```python
from build123d import *

# Parameters (mm, degrees)
SKETCH1_W                = 33.02
SKETCH1_H                = 10.16
SKETCH1_R                = 3
SKETCH1_R_2              = 1.7
BOSS_EXTRUDE1_DEPTH      = 1
SKETCH2_W                = 6
SKETCH2_H                = 1
SKETCH2_W_2              = 1
SKETCH2_H_2              = 6
BOSS_EXTRUDE2_DEPTH      = 6
SKETCH3_R                = 1
CUT_EXTRUDE1_DEPTH       = 21.610815122
FILLET1_R                = 1
BOSS_EXTRUDE3_DEPTH      = 1
BOSS_EXTRUDE3_DEPTH_BACK = 1


with BuildPart() as part:
    # Sketch1 → Boss-Extrude1 (new body)
    with BuildSketch(Plane(origin=(0, 0, 0), x_dir=(1, 0, 0), z_dir=(0, 1, 0))):
        Rectangle(SKETCH1_W, SKETCH1_H)
        with Locations(Location((0, 0, 0), (0, 0, 270))):
            Circle(SKETCH1_R, mode=Mode.SUBTRACT)
        with Locations(Location((-12.7, 0, 0), (0, 0, 270))):
            Circle(SKETCH1_R_2, mode=Mode.SUBTRACT)
    extrude(amount=BOSS_EXTRUDE1_DEPTH)

    # Sketch2 → Boss-Extrude2 (add)
    with BuildSketch(Plane(origin=(0, 1, 0), x_dir=(1, 0, 0), z_dir=(0, 1, 0))):
        with Locations((-12.7, 4.58)):
            Rectangle(SKETCH2_W, SKETCH2_H)
        with Locations((-12.7, -4.58)):
            Rectangle(SKETCH2_W, SKETCH2_H)
        with Locations((16.01, 0)):
            Rectangle(SKETCH2_W_2, SKETCH2_H_2)
    extrude(amount=BOSS_EXTRUDE2_DEPTH)

    # Sketch3 → Cut-Extrude1 (cut, through all)
    with BuildSketch(Plane.XY.offset(5.08)):
        with Locations((-12.7, 5)):
            Circle(SKETCH3_R)
    extrude(amount=-CUT_EXTRUDE1_DEPTH, mode=Mode.SUBTRACT)

    # Fillet1
    # the kernel refuses this fillet: 1 mm, written as the material it adds along each edge
    with BuildSketch(Plane(origin=(-15.7, 1, -4.08), x_dir=(-1, 0, 0), z_dir=(0, 0, -1))) as fillet1_piece_1:
        with BuildLine():
            CenterArc((1, 0.98178409), FILLET1_R, 180, 79.047215801)
            Line((0, 0.98178409), (0, 0))
            Line((0, 0), (0.81, 0))
        make_face()
    extrude(amount=1)
    with BuildSketch(Plane(origin=(-9.7, 1, -4.08), x_dir=(0, 0, 1), z_dir=(-1, 0, 0))) as fillet1_piece_2:
        with BuildLine():
            CenterArc((FILLET1_R, FILLET1_R), FILLET1_R, 180, 90)
            Line((0, FILLET1_R), (0, 0))
            Line((0, 0), (FILLET1_R, 0))
        make_face()
    extrude(amount=6)
    with BuildSketch(Plane(origin=(-9.7, 1, -5.08), x_dir=(1, 0, 0), z_dir=(0, 0, 1))) as fillet1_piece_3:
        with BuildLine():
            CenterArc((FILLET1_R, FILLET1_R), FILLET1_R, 180, 90)
            Line((0, FILLET1_R), (0, 0))
            Line((0, 0), (FILLET1_R, 0))
        make_face()
    extrude(amount=1)
    with BuildSketch(Plane(origin=(16.51, 1, -3), x_dir=(0, 0, -1), z_dir=(-1, 0, 0)), Plane(origin=(15.51, 1, 3), x_dir=(0, 0, 1), z_dir=(1, 0, 0)), Plane(origin=(-9.7, 1, 5.08), x_dir=(1, 0, 0), z_dir=(0, 0, -1))) as fillet1_piece_4:
        with BuildLine():
            CenterArc((FILLET1_R, -FILLET1_R), FILLET1_R, 90, 90)
            Line((0, -FILLET1_R), (0, 0))
            Line((0, 0), (FILLET1_R, 0))
        make_face()
    extrude(amount=1)
    with BuildSketch(Plane(origin=(-15.7, 1, 4.08), x_dir=(-1, 0, 0), z_dir=(0, 0, 1))) as fillet1_piece_5:
        with BuildLine():
            CenterArc((1, -0.98178409), FILLET1_R, 100.952784199, 79.047215801)
            Line((0, -0.98178409), (0, 0))
            Line((0, 0), (0.81, 0))
        make_face()
    extrude(amount=1)
    with BuildSketch(Plane(origin=(-9.7, 1, 4.08), x_dir=(0, 0, -1), z_dir=(-1, 0, 0))) as fillet1_piece_6:
        with BuildLine():
            CenterArc((FILLET1_R, -FILLET1_R), FILLET1_R, 90, 90)
            Line((0, -FILLET1_R), (0, 0))
            Line((0, 0), (FILLET1_R, 0))
        make_face()
    extrude(amount=6)
    with BuildSketch(Plane(origin=(-15.7, 1, -1.625539774), x_dir=(-1, 0, 0), z_dir=(0, 0, -1))) as fillet1_piece_7a_section:
        with BuildLine():
            CenterArc((1, 0.98178409), FILLET1_R, 180, 79.047215801)
            Line((0, 0.98178409), (0, 0))
            Line((0, 0), (0.81, 0))
        make_face()
    fillet1_piece_7a = extrude(amount=3.454460226, mode=Mode.PRIVATE)
    fillet1_piece_7a = split(fillet1_piece_7a, bisect_by=Plane(origin=(-15.7, 1, -4.08), z_dir=(0, 0, 1)), keep=Keep.TOP, mode=Mode.PRIVATE)
    with BuildSketch(Plane(origin=(-9.7, 1, -4.08), x_dir=(0, 0, 1), z_dir=(-1, 0, 0))) as fillet1_piece_7b_section:
        with BuildLine():
            CenterArc((FILLET1_R, FILLET1_R), FILLET1_R, 180, 90)
            Line((0, FILLET1_R), (0, 0))
            Line((0, 0), (FILLET1_R, 0))
        make_face()
    fillet1_piece_7b = extrude(amount=8.5, mode=Mode.PRIVATE)
    fillet1_piece_7b = split(fillet1_piece_7b, bisect_by=Plane(origin=(-16.51, 1, -4.08), z_dir=(1, 0, 0)), keep=Keep.TOP, mode=Mode.PRIVATE)
    fillet1_piece_7b = split(fillet1_piece_7b, bisect_by=Plane(origin=(-15.7, 1, -4.08), z_dir=(-1, 0, 0)), keep=Keep.TOP, mode=Mode.PRIVATE)
    fillet1_piece_7 = fillet1_piece_7a & fillet1_piece_7b
    add(fillet1_piece_7)
    with BuildSketch(Plane(origin=(-7.2, 1, -4.08), x_dir=(0, 0, 1), z_dir=(-1, 0, 0))) as fillet1_piece_8a_section:
        with BuildLine():
            CenterArc((FILLET1_R, FILLET1_R), FILLET1_R, 180, 90)
            Line((0, FILLET1_R), (0, 0))
            Line((0, 0), (FILLET1_R, 0))
        make_face()
    fillet1_piece_8a = extrude(amount=8.5, mode=Mode.PRIVATE)
    fillet1_piece_8a = split(fillet1_piece_8a, bisect_by=Plane(origin=(-9.7, 1, -4.08), z_dir=(1, 0, 0)), keep=Keep.TOP, mode=Mode.PRIVATE)
    with BuildSketch(Plane(origin=(-9.7, 1, -5.08), x_dir=(1, 0, 0), z_dir=(0, 0, 1))) as fillet1_piece_8b_section:
        with BuildLine():
            CenterArc((FILLET1_R, FILLET1_R), FILLET1_R, 180, 90)
            Line((0, FILLET1_R), (0, 0))
            Line((0, 0), (FILLET1_R, 0))
        make_face()
    fillet1_piece_8b = extrude(amount=3.5, mode=Mode.PRIVATE)
    fillet1_piece_8b = split(fillet1_piece_8b, bisect_by=Plane(origin=(-9.7, 1, -4.08), z_dir=(0, 0, 1)), keep=Keep.TOP, mode=Mode.PRIVATE)
    fillet1_piece_8 = fillet1_piece_8a & fillet1_piece_8b
    add(fillet1_piece_8)
    with BuildSketch(Plane(origin=(-9.7, 1, 4.08), x_dir=(0, 0, -1), z_dir=(-1, 0, 0))) as fillet1_piece_9a_section:
        with BuildLine():
            CenterArc((FILLET1_R, -FILLET1_R), FILLET1_R, 90, 90)
            Line((0, -FILLET1_R), (0, 0))
            Line((0, 0), (FILLET1_R, 0))
        make_face()
    fillet1_piece_9a = extrude(amount=8.5, mode=Mode.PRIVATE)
    fillet1_piece_9a = split(fillet1_piece_9a, bisect_by=Plane(origin=(-16.51, 1, 4.08), z_dir=(1, 0, 0)), keep=Keep.TOP, mode=Mode.PRIVATE)
    fillet1_piece_9a = split(fillet1_piece_9a, bisect_by=Plane(origin=(-15.7, 1, 4.08), z_dir=(-1, 0, 0)), keep=Keep.TOP, mode=Mode.PRIVATE)
    with BuildSketch(Plane(origin=(-15.7, 1, 1.625539774), x_dir=(-1, 0, 0), z_dir=(0, 0, 1))) as fillet1_piece_9b_section:
        with BuildLine():
            CenterArc((1, -0.98178409), FILLET1_R, 100.952784199, 79.047215801)
            Line((0, -0.98178409), (0, 0))
            Line((0, 0), (0.81, 0))
        make_face()
    fillet1_piece_9b = extrude(amount=3.454460226, mode=Mode.PRIVATE)
    fillet1_piece_9b = split(fillet1_piece_9b, bisect_by=Plane(origin=(-15.7, 1, 4.08), z_dir=(0, 0, -1)), keep=Keep.TOP, mode=Mode.PRIVATE)
    fillet1_piece_9 = fillet1_piece_9a & fillet1_piece_9b
    add(fillet1_piece_9)
    with BuildSketch(Plane(origin=(-9.7, 1, 5.08), x_dir=(1, 0, 0), z_dir=(0, 0, -1))) as fillet1_piece_10a_section:
        with BuildLine():
            CenterArc((FILLET1_R, -FILLET1_R), FILLET1_R, 90, 90)
            Line((0, -FILLET1_R), (0, 0))
            Line((0, 0), (FILLET1_R, 0))
        make_face()
    fillet1_piece_10a = extrude(amount=3.5, mode=Mode.PRIVATE)
    fillet1_piece_10a = split(fillet1_piece_10a, bisect_by=Plane(origin=(-9.7, 1, 4.08), z_dir=(0, 0, -1)), keep=Keep.TOP, mode=Mode.PRIVATE)
    with BuildSketch(Plane(origin=(-7.2, 1, 4.08), x_dir=(0, 0, -1), z_dir=(-1, 0, 0))) as fillet1_piece_10b_section:
        with BuildLine():
            CenterArc((FILLET1_R, -FILLET1_R), FILLET1_R, 90, 90)
            Line((0, -FILLET1_R), (0, 0))
            Line((0, 0), (FILLET1_R, 0))
        make_face()
    fillet1_piece_10b = extrude(amount=8.5, mode=Mode.PRIVATE)
    fillet1_piece_10b = split(fillet1_piece_10b, bisect_by=Plane(origin=(-9.7, 1, 4.08), z_dir=(1, 0, 0)), keep=Keep.TOP, mode=Mode.PRIVATE)
    fillet1_piece_10 = fillet1_piece_10a & fillet1_piece_10b
    add(fillet1_piece_10)
    # the kernel refuses this fillet: 1 mm, written as the material it takes off along each edge
    with BuildSketch(Plane(origin=(-15.7, 7, -1.58), x_dir=(0, -1, 0), z_dir=(0, 0, -1)), Plane(origin=(13.01, 7, 3), x_dir=(0, 0, -1), z_dir=(1, 0, 0)), Plane(origin=(-15.7, 7, 1.58), x_dir=(1, 0, 0), z_dir=(0, 0, 1)), Plane(origin=(16.51, -2.5, 5.08), x_dir=(-1, 0, 0), z_dir=(0, 1, 0))) as fillet1_2_piece_1:
        with BuildLine():
            CenterArc((FILLET1_R, -FILLET1_R), FILLET1_R, 90, 90)
            Line((0, -FILLET1_R), (0, 0))
            Line((0, 0), (FILLET1_R, 0))
        make_face()
    extrude(amount=6, mode=Mode.SUBTRACT)
    with BuildSketch(Plane(origin=(-9.7, 7, -7.58), x_dir=(-1, 0, 0), z_dir=(0, 0, 1)), Plane(origin=(19.01, 7, -3), x_dir=(0, -1, 0), z_dir=(-1, 0, 0)), Plane(origin=(-9.7, 7, 7.58), x_dir=(0, -1, 0), z_dir=(0, 0, -1)), Plane(origin=(16.51, -2.5, -5.08), x_dir=(-1, 0, 0), z_dir=(0, 1, 0))) as fillet1_2_piece_2:
        with BuildLine():
            CenterArc((FILLET1_R, FILLET1_R), FILLET1_R, 180, 90)
            Line((0, FILLET1_R), (0, 0))
            Line((0, 0), (FILLET1_R, 0))
        make_face()
    extrude(amount=6, mode=Mode.SUBTRACT)

    # Sketch4 → Boss-Extrude3 (add, two sides: drawn at the far end of the back side and taken through both)
    with BuildSketch(Plane.XY.offset(-BOSS_EXTRUDE3_DEPTH_BACK)):
        Polygon((14.51, 5), (15.51, 6), (15.51, 4.5), (14.51, 4.5), align=None)
    extrude(amount=BOSS_EXTRUDE3_DEPTH + BOSS_EXTRUDE3_DEPTH_BACK)


solid = part.part
```
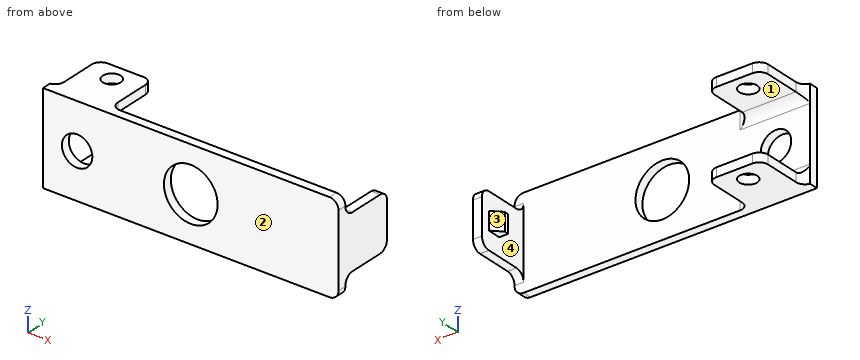
Here's how the part is built. I have some questions about the finished solid (model axes, mm). Face numbers are marked on the shaded views. Coordinates: 2 decimals unless noted, no trailing zeros. Order: outer loops, then holes, each group sorted by start corner. A loop starts at its lowest first (then second) coordinate and runs counter-clockwise, first axis right, second up.
1) Imagine slicing it at B-B on x = -12.7. List the corners of the cut face in (y, z) for me.
2) Imagine slicing it at A-A on y = 3.25. List the corners of the cut face in (x, z) for me, and give its area (3 significant figures).
3) Will these pins go through, and if not, where does the flat tip stop? pin 1 (4 mm diameter, centred on x = -6, z = 1, fed in from +Y); pin 2 (0.8 mm diameter, centred on x = 15, y = 5, fed in from +Z); pin 3 (0.8 mm diameter, centred on y = 5, z = 4.5, fed in from +X).
4) We'd pull the mould along Y, two halves only. Please class the marked faces 1, 2, 3 and 4: +Y half, -Y half, draft (parallel to the pull), parting line (faces both ways), or undercut.
5) Imagine slicing it at C-C on z = 0. List the corners of the cut face in (x, y) for me.
6) Imagine slicing it at D-D on x = 0. List the corners of the cut face in (y, z) for me, and give its area (3 significant figures).
7) I need wall thicknesses on line 1 (Y direction, x = -12.7, z = 4.5); line 2 (Y direction, x = -12, z = -3); line 3 (X direction, y = 6, z = 2.5). Which ranges of each line are inside material? Lowest first, please.
Response values:
1. outline: (0, -5.08) - (4, -5.08) - (4, -4.08) - (2, -4.08) arc R1 cw to (1, -3.08) - (1, -1.7) - (0, -1.7) - close; (0, 1.7) - (1, 1.7) - (1, 3.08) arc R1 cw to (2, 4.08) - (4, 4.08) - (4, 5.08) - (0, 5.08) - close; (6, -5.08) - (7, -5.08) - (7, -4.08) - (6, -4.08) - close; (6, 4.08) - (7, 4.08) - (7, 5.08) - (6, 5.08) - close
2. outline: (-15.7, -5.08) - (-9.7, -5.08) - (-9.7, -4.08) - (-15.7, -4.08) - close; (-15.7, 4.08) - (-9.7, 4.08) - (-9.7, 5.08) - (-15.7, 5.08) - close; (15.51, -3) - (16.51, -3) - (16.51, 3) - (15.51, 3) - close
2. area: 18.0 mm2
3. pin 1: stops at y = 1
3. pin 2: stops at z = 1
3. pin 3: stops at x = -9.7
4. face 1: draft
4. face 2: -Y half
4. face 3: +Y half
4. face 4: undercut
5. outline: (-16.51, 0) - (-14.4, 0) - (-14.4, 1) - (-16.51, 1) - close; (-11, 0) - (-3, 0) - (-3, 1) - (-11, 1) - close; (3, 0) - (16.51, 0) - (16.51, 7) - (15.51, 7) - (15.51, 6) - (14.51, 5) - (14.51, 4.5) - (15.51, 4.5) - (15.51, 1) - (3, 1) - close
6. outline: (0, -5.08) - (1, -5.08) - (1, -3) - (0, -3) - close; (0, 3) - (1, 3) - (1, 5.08) - (0, 5.08) - close
6. area: 4.16 mm2
7. line 1: y = 0 to 4, 6 to 7
7. line 2: y = 0 to 1
7. line 3: x = 15.51 to 16.51
